from build123d import *

# Parameters (mm, degrees)
ESQUISSE1_R                  = 21.4
BOSS_EXTRU_1_DEPTH           = 10
ESQUISSE2_R                  = 25
BOSS_EXTRU_2_DEPTH           = 2
ENL_V_MAT_EXTRU_1_DEPTH      = 38.336309405
ENL_V_MAT_EXTRU_1_DEPTH_BACK = 38.336309405
ESQUISSE3_R                  = 4.2
CHANFREIN1_SIZE              = 1


with BuildPart() as part:
    # Esquisse1 → Boss.-Extru.1 (new body)
    with BuildSketch(Plane.XY):
        Circle(ESQUISSE1_R)
    extrude(amount=BOSS_EXTRU_1_DEPTH)

    # Esquisse2 → Boss.-Extru.2 (add)
    with BuildSketch(Plane.XY.offset(10)):
        Circle(ESQUISSE2_R)
    extrude(amount=BOSS_EXTRU_2_DEPTH)

    # Esquisse3 → Enlèv. mat.-Extru.1 (cut, two sides: drawn at the far end of the back side and taken through both)
    with BuildSketch(Plane.XY.offset(12).offset(-ENL_V_MAT_EXTRU_1_DEPTH_BACK)):
        Circle(ESQUISSE3_R)
    extrude(amount=ENL_V_MAT_EXTRU_1_DEPTH + ENL_V_MAT_EXTRU_1_DEPTH_BACK, mode=Mode.SUBTRACT)

    # Chanfrein1
    chanfrein1_edges = [part.edges().sort_by_distance(p)[0] for p in [
        (-4.2, 0, 12),
        (-4.2, 0, 0),
        (-21.4, 0, 0),
    ]]
    chamfer(chanfrein1_edges, length=CHANFREIN1_SIZE)


solid = part.part
Work out the finished part from the listing and answer in its coordinate system (mm). A direction names the side the tool comes from. Give positions to 0.01 mm unless a question says otherwise; leave off trailing zeros. Write each loop counter-clockwise with the first axis right and the second up, starting at its lowest first coordinate (ties: lowest second). Pieces come first, ordered by that corner, then holes.
Q1. The part is cut by section D-D on y = -22. Give the vertices of the cut face in (x, z).
Answer:
outline: (-11.87, 10) - (11.87, 10) - (11.87, 12) - (-11.87, 12) - close
Q2. Given pin 1 (5 mm diameter, centred on x = -18.5, z = 5, fed in from +Y); pin 2 (6 mm diameter, centred on y = -6, z = 4, fed in from +X); pin 3 (5 mm diameter, centred on x = -0.5, z = 8, fed in from +Y), each flat-ended and moving along its own axis, determine where each tip first touches the part or whether it passes through.
Answer:
pin 1: stops at y = 14.21
pin 2: stops at x = 21.19
pin 3: stops at y = 25
Q3. A tool of negligible diameter and unlimited length cuts with its end or side. For faces 1 (the face through (4, -4, 0)), 2 (the face through (18.4, 11.23, 10)), from which of +Z, -Z, +X, -X, +Y, -Y can it reach the whole face along a straight path? Write none if from no direction.
Answer:
face 1: -Z, +X, -X, +Y, -Y
face 2: -Z
Q4. The part is cut by section A-A on x = 0. Give the vertices of the cut face in (y, z).
Answer:
outline: (-25, 10) - (-21.4, 10) - (-21.4, 1) - (-20.4, 0) - (-5.2, 0) - (-4.2, 1) - (-4.2, 11) - (-5.2, 12) - (-25, 12) - close; (4.2, 1) - (5.2, 0) - (20.4, 0) - (21.4, 1) - (21.4, 10) - (25, 10) - (25, 12) - (5.2, 12) - (4.2, 11) - close
Q5. Straight lines are drawn through the part: L1, parallel to Y at x = 0, z = 7.75; L2, parallel to Z at x = -4, y = -21.5; L3, parallel to X at y = -3.5, z = 1.75. For each, find the intervals that lie inside material, in ascending order.
Answer:
L1: y = -21.4 to -4.2, 4.2 to 21.4
L2: z = 10 to 12
L3: x = -21.11 to -2.32, 2.32 to 21.11
Q6. For a pull along Y with two mould halves and no side action, classify faces 3 (the face through (0, 6, 12)), 4 (the face through (23.846, 7.509, 10.986)), 5 (the face through (4.006, 1.262, 5.93)) as released by +Y, released by -Y, zero draft, split by the parting line, or undercut.
Answer:
face 3: zero draft
face 4: split by the parting line
face 5: undercut
Q7. The part is cut by section C-C on z = 4.5. Give the vertices of the cut face in (x, y).
Answer:
outline: circle Ø42.8 at (0, 0); hole circle Ø8.4 at (0, 0)
